```python
from build123d import *

# Parameters (mm, degrees)
F0_W     = 25.4
F0_H     = 3.302
F1_DEPTH = 3.302
F2_R     = 1
F3_DEPTH = 5.08
F4_R     = 0.9525


with BuildPart() as f1:
    # F0 (on Top) → F1 (new body)
    with BuildSketch(Plane.XY):
        with Locations((12.7, 1.651)):
            Rectangle(F0_W, F0_H)
    extrude(amount=F1_DEPTH)

    # F2 (on face) → F3 (cut)
    with BuildSketch(Plane(origin=(0, 0, 0), x_dir=(0, -1, 0), z_dir=(-1, 0, 0))):
        with Locations((-1.651, 1.651)):
            Circle(F2_R)
    extrude(amount=-F3_DEPTH, mode=Mode.SUBTRACT)

    # F7: sweep along a path in F6
    with BuildLine(Plane.XZ.offset(-1.651)) as f7_path:
        ThreePointArc((23.749, 3.302), (24.2325667043, 2.1345667043), (25.4, 1.651))
    # F4 (on face) → F7 (sweep, cut)
    with BuildSketch(Plane.YZ.offset(25.4)):
        with Locations((1.651, 1.651)):
            Circle(F4_R)
    sweep(path=f7_path.line, mode=Mode.SUBTRACT)


solid = f1.part
```
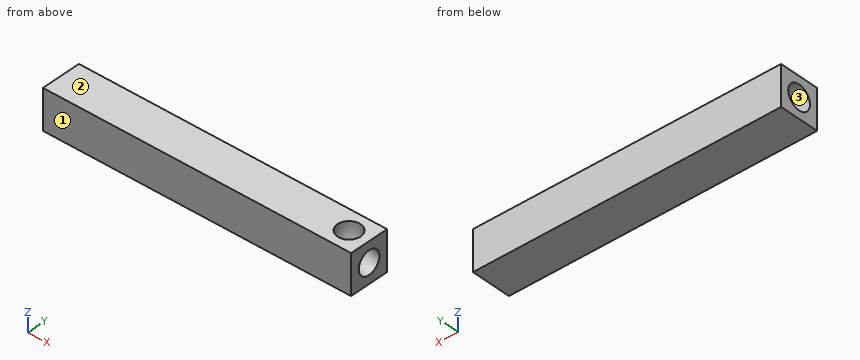
Design review of the part built by this model. Coordinates are the model's own, in mm. Face numbers are marked on the shaded views. Coordinates: 2 decimals unless noted, no trailing zeros. Order: outer loops, then holes, each group sorted by start corner. A loop starts at its lowest first (then second) coordinate and runs counter-clockwise, first axis right, second up.
1) Clearance check with a flat-ended pin moving along its axis: pin 1 (1 mm diameter, centred on x = 8, z = 1.5, fed in from -Y). State where the tip first meets the part, or that it passes through.
2) Mouldability with a two-part tool opening along Z and no side actions: class the marked faces 1, 2 and 3 as +Z half, -Z half, draft (parallel to the pull), parting line (faces both ways), or undercut.
3) Take a section at A-A, the plane y = 1.15. Give the boundary of the cut face in (x, z), and give its area (3 significant figures).
4) Take a section at B-B, the plane x = 4. Give the boundary of the cut face in (y, z), and give its area (3 significant figures).
5) Wall thickness on line 1 along Y through (x, z) = (1.5, 2.3); line 2 along X through (y, z) = (2.5, 2.9); line 3 along Z through (x, y) = (2, 0.85): over which ranges is each line inside the solid? List them lowest first.
Returned:
1. pin 1: stops at y = 0
2. face 1: draft
2. face 2: +Z half
2. face 3: undercut
3. outline: (0, 0) - (25.4, 0) - (25.4, 0.84) arc R2.46 cw to (22.94, 3.3) - (0, 3.3) - (0, 2.52) - (5.08, 2.52) - (5.08, 0.79) - (0, 0.79) - close; (24.56, 3.3) arc R0.84 ccw to (25.4, 2.46) - (25.4, 3.3) - close
3. area: 70.9 mm2
4. outline: (0, 0) - (3.3, 0) - (3.3, 3.3) - (0, 3.3) - close; hole circle Ø2 at (1.65, 1.65)
4. area: 7.76 mm2
5. line 1: y = 0 to 0.89, 2.41 to 3.3
5. line 2: x = 0 to 23.36, 24.25 to 25.4
5. line 3: z = 0 to 1.05, 2.25 to 3.3
